Work out the finished part from the listing and answer in its coordinate system (mm). Round coordinates to 2 decimals unless told otherwise and drop trailing zeros. Order: outer loops, then holes, each group sorted by start corner. A loop starts at its lowest first (then second) coordinate and runs counter-clockwise, first axis right, second up. Notation, with made-up numbers: (66.25, 21) - (97.25, 21) arc R14 cw to (97.25, 28) - close; hole circle Ø2 at (73.25, 20.5). An arc over 180 degrees is marked (long way). Put each result on its own line as item: value.
```python
from build123d import *

# Parameters (mm, degrees)
SKETCH2_R           = 63.2206
SKETCH2_R_2         = 3.175
SKETCH2_R_3         = 1.8288
BOSS_EXTRUDE1_DEPTH = 3.175


with BuildPart() as part:
    # Sketch2 → Boss-Extrude1 (new body)
    with BuildSketch(Plane(origin=(0, 0, 0), x_dir=(1, 0, 0), z_dir=(0, 1, 0))):
        Circle(SKETCH2_R)
        with Locations((-46.99, 0)):
            Circle(SKETCH2_R_2, mode=Mode.SUBTRACT)
        with Locations((46.99, 0)):
            Circle(SKETCH2_R_2, mode=Mode.SUBTRACT)
        Circle(SKETCH2_R_2, mode=Mode.SUBTRACT)
        with Locations((0, 38.1)):
            Circle(SKETCH2_R_3, mode=Mode.SUBTRACT)
        with Locations((0, -38.1)):
            Circle(SKETCH2_R_3, mode=Mode.SUBTRACT)
        with Locations((-26.940768363, 26.940768363)):
            Circle(SKETCH2_R_3, mode=Mode.SUBTRACT)
        with Locations((26.940768363, -26.940768363)):
            Circle(SKETCH2_R_3, mode=Mode.SUBTRACT)
    extrude(amount=BOSS_EXTRUDE1_DEPTH)


solid = part.part
```
1) Straight lines are drawn through the part: L1, parallel to X at y = 2, z = -38.1; L2, parallel to X at y = 2.9, z = -1; L3, parallel to X at y = 1.4, z = 49.5. For each, find the intervals that lie inside material, in ascending order. Write a range as from..to.
Findings below:
L1: x = -50.45..-1.83, 1.83..50.45
L2: x = -63.21..-50, -43.98..-3.01, 3.01..43.98, 50..63.21
L3: x = -39.33..39.33
2) A cutting plane is placed at A-A on x = 0. Write down the section's boundary in (y, z) (3 decimals), then the cut area to 3 significant figures.
Findings below:
outline: (0, -63.221) - (3.175, -63.221) - (3.175, -39.929) - (0, -39.929) - close; (0, -36.271) - (3.175, -36.271) - (3.175, -3.175) - (0, -3.175) - close; (0, 3.175) - (3.175, 3.175) - (3.175, 36.271) - (0, 36.271) - close; (0, 39.929) - (3.175, 39.929) - (3.175, 63.221) - (0, 63.221) - close
area: 358 mm2
3) A cutting plane is placed at D-D on x = 46.99. Write down the section's boundary in (y, z) (3 decimals).
Findings below:
outline: (0, -42.294) - (3.175, -42.294) - (3.175, -3.175) - (0, -3.175) - close; (0, 3.175) - (3.175, 3.175) - (3.175, 42.294) - (0, 42.294) - close
4) A cutting plane is placed at C-C on z = -38.1. Write down the section's boundary in (x, y) (3 decimals), then the cut area to 3 significant figures.
Findings below:
outline: (-50.45, 0) - (-1.829, 0) - (-1.829, 3.175) - (-50.45, 3.175) - close; (1.829, 0) - (50.45, 0) - (50.45, 3.175) - (1.829, 3.175) - close
area: 309 mm2
5) A cutting plane is placed at B-B on z = 0. Write down the section's boundary in (x, y) (3 decimals).
Findings below:
outline: (-63.221, 0) - (-50.165, 0) - (-50.165, 3.175) - (-63.221, 3.175) - close; (-43.815, 0) - (-3.175, 0) - (-3.175, 3.175) - (-43.815, 3.175) - close; (3.175, 0) - (43.815, 0) - (43.815, 3.175) - (3.175, 3.175) - close; (50.165, 0) - (63.221, 0) - (63.221, 3.175) - (50.165, 3.175) - close
6) Given pin 1 Ø5.5 at (x, z) = (0, 0) entering from +Y; pin 2 Ø1 at (x, y) = (7.5, 1) entering from -Z, each flat-ended and moving along its own axis, determine where each tip first touches the part or whether it passes through.
Findings below:
pin 1: passes through
pin 2: stops at z = -62.83
7) For a pull along X with two mould halves and no side action, classify faces 1 (the cylindrical face through (-8.23, 1.565, -62.683)), 2 (the flat face through (13, 0, -1)), 3 (the cylindrical face through (50.02, 1.57, -0.95)) as pulls with the +X half, pulls with the -X half, needs draft (parallel to the pull), parting line crosses it, or undercut.
Findings below:
face 1: parting line crosses it
face 2: needs draft
face 3: undercut
